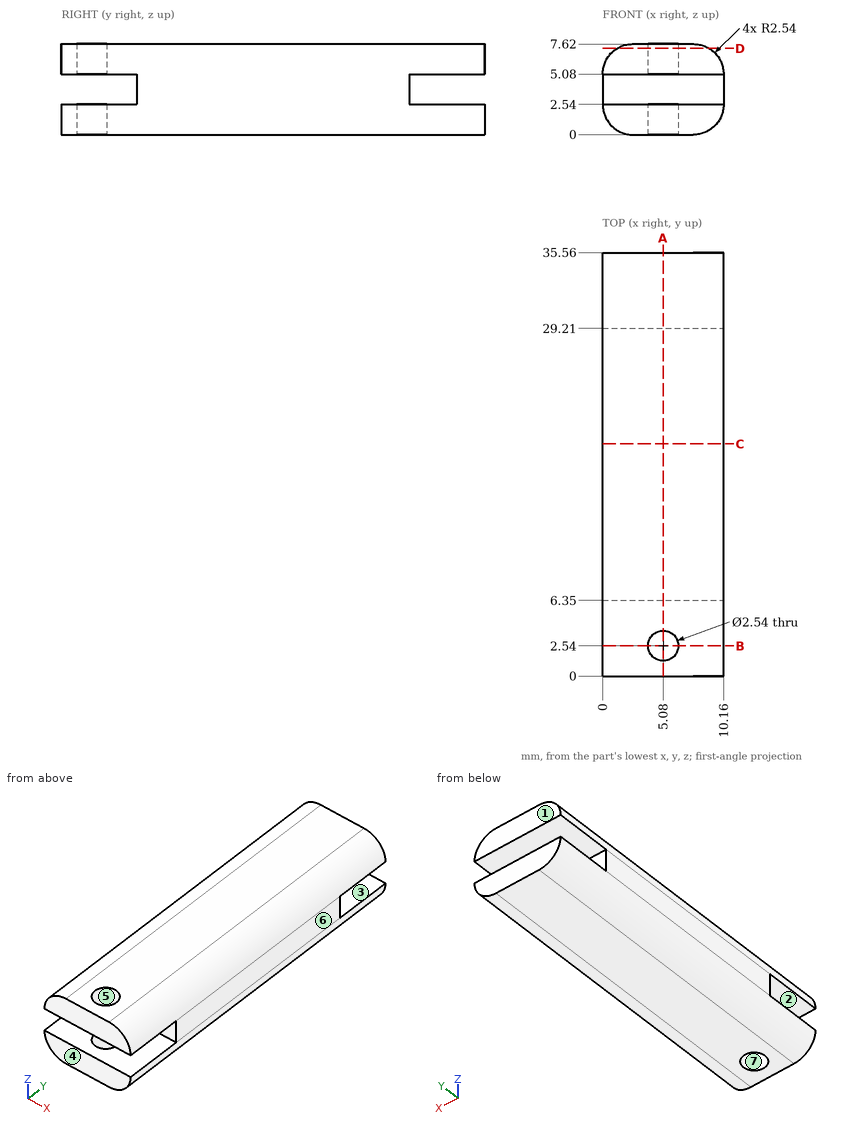
Study the drawing (mm; zero at the part's minimum x, y, z) and answer. A direction names the side the tool comes from. Round coordinates to 2 decimals unless told otherwise and drop trailing zeros. Loops run counter-clockwise (first coordinate to the right, second up) from the corner with the lowest first, then second, coordinate; pieces in that order, holes last.
Q1. Section D-D, the plane z = 7.25 is taken. Determine the outline of the cut face in (x, y), then the cut area to 3 significant figures.
Q2. Section A-A, the plane x = 5.08 is taken. Determine the outline of the cut face in (y, z).
Q3. For a pull along X with two mould halves and no side action, classify the marked faces 4, 5, 6 and 7 as released by +X, released by -X, zero draft, split by the parting line, or undercut.
Q4. Section C-C, the plane y = 19.5 is taken. Determine the outline of the cut face in (x, z), then the cut area to 3 significant figures.
Q5. Given pin 1 Ø4 at (x, y) = (1.5, 7) entering from -Z, flat-ended and moving along its own axis, determine where the tip first touches the part or whether it passes through.
Q6. Section B-B, the plane y = 2.54 is taken. Determine the outline of the cut face in (x, z), then the cut area to 3 significant figures.
Q7. Find the intervals of material crossed by line 1 (Y direction, x = 5.08, z = 6.7); line 2 (Z direction, x = 3.75, y = 33.5); line 3 (X direction, y = 3, z = 6.75), in increasing order.
Q8. Which of the six approach directions +Z, -Z, +X, -X, +Y, -Y give full straight-line access (tool end or side, diameter ignored) to the marked faces 1, 2 and 3?
Completed:
1. outline: (1.22, 0) - (8.94, 0) - (8.94, 35.56) - (1.22, 35.56) - close; hole circle Ø2.54 at (5.08, 2.54)
1. area: 269 mm2
2. outline: (0, 0) - (1.27, 0) - (1.27, 2.54) - (0, 2.54) - close; (0, 5.08) - (1.27, 5.08) - (1.27, 7.62) - (0, 7.62) - close; (3.81, 0) - (35.56, 0) - (35.56, 2.54) - (29.21, 2.54) - (29.21, 5.08) - (35.56, 5.08) - (35.56, 7.62) - (3.81, 7.62) - (3.81, 5.08) - (6.35, 5.08) - (6.35, 2.54) - (3.81, 2.54) - close
3. face 4: zero draft
3. face 5: undercut
3. face 6: released by +X
3. face 7: undercut
4. outline: (0, 2.54) arc R2.54 ccw to (2.54, 0) - (7.62, 0) arc R2.54 ccw to (10.16, 2.54) - (10.16, 5.08) arc R2.54 ccw to (7.62, 7.62) - (2.54, 7.62) arc R2.54 ccw to (0, 5.08) - close
4. area: 71.9 mm2
5. pin 1: stops at z = 0
6. outline: (0, 2.54) arc R2.54 ccw to (2.54, 0) - (3.81, 0) - (3.81, 2.54) - close; (0, 5.08) - (3.81, 5.08) - (3.81, 7.62) - (2.54, 7.62) arc R2.54 ccw to start; (6.35, 0) - (7.62, 0) arc R2.54 ccw to (10.16, 2.54) - (6.35, 2.54) - close; (6.35, 5.08) - (10.16, 5.08) arc R2.54 ccw to (7.62, 7.62) - (6.35, 7.62) - close
6. area: 33.2 mm2
7. line 1: y = 0 to 1.27, 3.81 to 35.56
7. line 2: z = 0 to 2.54, 5.08 to 7.62
7. line 3: x = 0.63 to 3.9, 6.26 to 9.53
8. face 1: +Z, -Z, +X, -X, +Y
8. face 2: +X, -X, -Y
8. face 3: +X, -X, +Y
